```python
from build123d import *

# Parameters (mm, degrees)
SKETCH_3_R      = 2
SKETCH_3_R_2    = 1.999999997
SKETCH_3_R_3    = 1.999999995
SKETCH_3_R_4    = 1.5
EXTRUDE_1_DEPTH = 2


with BuildPart() as part:
    # 草图3 → 凸台-拉伸1 (new body)
    with BuildSketch(Plane.XY):
        with BuildLine():
            Line((-25.9, -3.990216685), (-25.9, 0.109783315))
            Line((-25.9, 0.109783315), (-15.9, 0.109783315))
            Line((-15.9, 0.109783315), (-6.948981504, 0.109783315))
            Line((-6.948981504, 0.109783315), (-6.948981504, 4.809783315))
            Line((-6.948981504, 4.809783315), (6.948981504, 4.809783315))
            Line((6.948981504, 4.809783315), (6.948981504, 0.109783315))
            Line((6.948981504, 0.109783315), (15.9, 0.109783315))
            Line((15.9, 0.109783315), (25.9, 0.109783315))
            Line((25.9, 0.109783315), (25.9, -3.990216685))
            Line((25.9, -3.990216685), (25.9, -4.990216685))
            Line((25.9, -4.990216685), (45, -4.990216685))
            Line((45, -4.990216685), (45, -3.990216685))
            Line((45, -3.990216685), (45, 8.890084071))
            Line((45, 8.890084071), (45, 21.128606731))
            Line((45, 21.128606731), (45, 31.317051182))
            ThreePointArc((45, 31.317051182), (36.482419799, 34.124770496), (28.474223712, 30.087289143))
            ThreePointArc((28.474223712, 30.087289143), (27.223611076, 28.776388924), (25.912710857, 27.525776288))
            ThreePointArc((25.912710857, 27.525776288), (15.928828372, 17.542283516), (1.809761925, 17.542559084))
            ThreePointArc((1.809761925, 17.542559084), (0, 17.5), (-1.809761925, 17.542559084))
            ThreePointArc((-1.809761925, 17.542559084), (-15.928828372, 17.542283516), (-25.912710857, 27.525776288))
            ThreePointArc((-25.912710857, 27.525776288), (-27.223611076, 28.776388924), (-28.474223712, 30.087289143))
            ThreePointArc((-28.474223712, 30.087289143), (-36.482419799, 34.124770496), (-45, 31.317051182))
            Line((-45, 31.317051182), (-45, 21.128606731))
            Line((-45, 21.128606731), (-45, 8.890084071))
            Line((-45, 8.890084071), (-45, -3.990216685))
            ThreePointArc((-45, -3.990216685), (-44.707106781, -4.697323466), (-44, -4.990216685))
            Line((-44, -4.990216685), (-25.9, -4.990216685))
            Line((-25.9, -4.990216685), (-25.9, -3.990216685))
        make_face()
        with Locations((0, 13.5)):
            Circle(SKETCH_3_R, mode=Mode.SUBTRACT)
        with Locations((-30.0520382, 25.94796181)):
            Circle(SKETCH_3_R_2, mode=Mode.SUBTRACT)
        with Locations((30.052038207, 25.947961792)):
            Circle(SKETCH_3_R_3, mode=Mode.SUBTRACT)
        with Locations((-23.174490752, 11.959783315)):
            Circle(SKETCH_3_R_4, mode=Mode.SUBTRACT)
        with Locations(Location((23.174490752, 11.959783315, 0), (0, 0, 180))):
            Circle(SKETCH_3_R_4, mode=Mode.SUBTRACT)
        with Locations((40.5, 15.059783315)):
            Circle(SKETCH_3_R_4, mode=Mode.SUBTRACT)
        with Locations(Location((-40.5, 15.059783315, 0), (0, 0, 180))):
            Circle(SKETCH_3_R_4, mode=Mode.SUBTRACT)
        with BuildLine():
            Line((-37.1, -2.090216685), (-29.9, -2.090216685))
            Line((-29.9, -2.090216685), (-29.9, 0.109783315))
            Line((-29.9, 0.109783315), (-37.1, 0.109783315))
            ThreePointArc((-37.1, 0.109783315), (-37.555634919, -0.990216685), (-37.1, -2.090216685))
        make_face(mode=Mode.SUBTRACT)
        with BuildLine():
            Line((-41.6, 25.109783315), (-39.4, 25.109783315))
            Line((-39.4, 25.109783315), (-39.4, 19.909783315))
            ThreePointArc((-39.4, 19.909783315), (-40.5, 19.454148396), (-41.6, 19.909783315))
            Line((-41.6, 19.909783315), (-41.6, 25.109783315))
        make_face(mode=Mode.SUBTRACT)
        with BuildLine():
            Line((-39.4, 10.109783315), (-39.4, 4.809783315))
            Line((-39.4, 4.809783315), (-41.6, 4.809783315))
            Line((-41.6, 4.809783315), (-41.6, 10.109783315))
            ThreePointArc((-41.6, 10.109783315), (-40.5, 10.565418233), (-39.4, 10.109783315))
        make_face(mode=Mode.SUBTRACT)
        with BuildLine():
            Line((37.1, 0.109783315), (29.9, 0.109783315))
            Line((29.9, 0.109783315), (29.9, -2.090216685))
            Line((29.9, -2.090216685), (37.1, -2.090216685))
            ThreePointArc((37.1, -2.090216685), (37.555634919, -0.990216685), (37.1, 0.109783315))
        make_face(mode=Mode.SUBTRACT)
        with BuildLine():
            Line((41.6, 4.809783315), (41.6, 10.109783315))
            ThreePointArc((41.6, 10.109783315), (40.5, 10.565418233), (39.4, 10.109783315))
            Line((39.4, 10.109783315), (39.4, 4.809783315))
            Line((39.4, 4.809783315), (41.6, 4.809783315))
        make_face(mode=Mode.SUBTRACT)
        with BuildLine():
            Line((39.4, 25.109783315), (39.4, 19.909783315))
            ThreePointArc((39.4, 19.909783315), (40.5, 19.454148396), (41.6, 19.909783315))
            Line((41.6, 19.909783315), (41.6, 25.109783315))
            Line((41.6, 25.109783315), (39.4, 25.109783315))
        make_face(mode=Mode.SUBTRACT)
    extrude(amount=EXTRUDE_1_DEPTH)


solid = part.part
```
Here's how the part is built. I have some questions about the finished solid (model axes, mm). A direction names the side the tool comes from. Coordinates: 2 decimals unless noted, no trailing zeros. Order: outer loops, then holes, each group sorted by start corner. A loop starts at its lowest first (then second) coordinate and runs counter-clockwise, first axis right, second up. Notation, with made-up numbers: (8, 62) - (17, 62) arc R28 ccw to (17, 82) - close; hole circle Ø11 at (57, -39). An arc over 180 degrees is marked (long way). One line per question, with ' | ' between items. Start each with the question number.
1. If we section it at D-D (y = 18.5): Write out the boundary of the cut face in (x, z), and give its area (3 significant figures).
2. If we section it at C-C (x = 0): Write out the boundary of the cut face in (y, z), and give its area (3 significant figures).
3. If we section it at B-B (x = 40.5): Write out the boundary of the cut face in (y, z).
4. I'm going to push flat-ended pins straight in: pin 1 Ø1 at (x, z) = (-14.5, 0.5) entering from -Y; pin 2 Ø1 at (x, z) = (-34.5, 1.5) entering from +Y. Where does each tip first touch, or does it pass through?
5. Please list where these lines run through material, in increasing order: line 1 along X through (y, z) = (9.5, 0.3); line 2 along X through (y, z) = (-1, 0.65); line 3 along X through (y, z) = (0, 0.25). Write a range as [from, to].
6. Which directions (+Z, -Z, +X, -X, +Y, -Y) give clear straight access to the entire face, cutting with the end or side of a thin tool? Please do faces 1 (the cylindrical face through (40.517, 10.565, 0.986)), 2 (the flat face through (-1, 11, 0)), 3 (the flat face through (-25.9, -2, 1)).
7. If we mould it in two halves opening along Y, with no side actions, what happens to faces 4 (the flat face through (-17, 0.11, 1)), 5 (the cylindrical face through (-37.556, -0.973, 0.986)), 6 (the flat face through (45, 13, 1)), 7 (the flat face through (-39.4, 23, 1))? For each: released by +Y, released by -Y, zero draft, split by the parting line, or undercut.
8. If we section it at A-A (y = 6): Write out the boundary of the cut face in (x, z), and give its area (3 significant figures).
Model answer:
1) outline: (-45, 0) - (-17.9, 0) - (-17.9, 2) - (-45, 2) - close; (17.9, 0) - (45, 0) - (45, 2) - (17.9, 2) - close | area: 108 mm²
2) outline: (4.81, 0) - (11.5, 0) - (11.5, 2) - (4.81, 2) - close; (15.5, 0) - (17.5, 0) - (17.5, 2) - (15.5, 2) - close | area: 17.4 mm²
3) outline: (-4.99, 0) - (4.81, 0) - (4.81, 2) - (-4.99, 2) - close; (10.57, 0) - (13.56, 0) - (13.56, 2) - (10.57, 2) - close; (16.56, 0) - (19.45, 0) - (19.45, 2) - (16.56, 2) - close; (25.11, 0) - (33.73, 0) - (33.73, 2) - (25.11, 2) - close
4) pin 1: stops at y = 0.11 | pin 2: stops at y = 33.92
5) line 1: x = [-45, -41.6], [-39.4, 39.4], [41.6, 45] | line 2: x = [-45, -37.56], [-29.9, -25.9], [25.9, 29.9], [37.56, 45] | line 3: x = [-45, -37.2], [-29.9, -25.9], [25.9, 29.9], [37.2, 45]
6) face 1: +Z, -Z | face 2: -Z, +X, -X, +Y, -Y | face 3: +Z, -Z, -Y
7) face 4: released by -Y | face 5: undercut | face 6: zero draft | face 7: undercut
8) outline: (-45, 0) - (-41.6, 0) - (-41.6, 2) - (-45, 2) - close; (-39.4, 0) - (39.4, 0) - (39.4, 2) - (-39.4, 2) - close; (41.6, 0) - (45, 0) - (45, 2) - (41.6, 2) - close | area: 171 mm²
